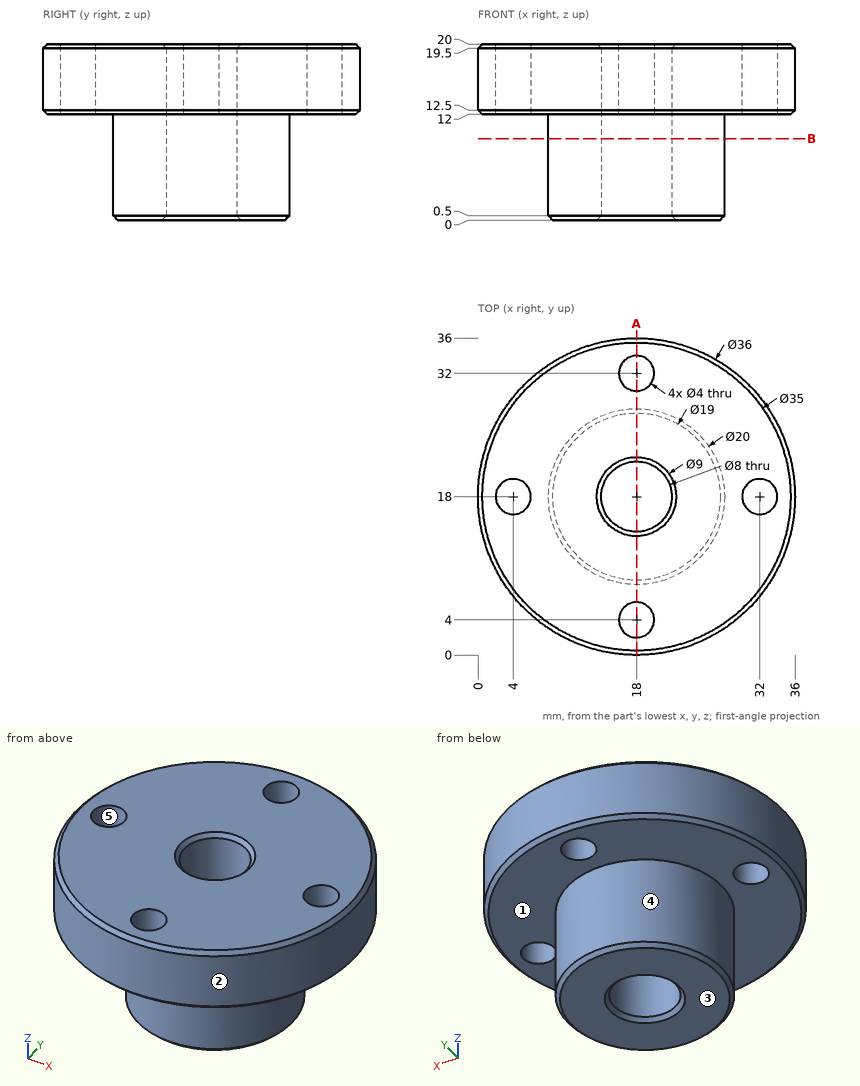
Part print with two shaded views. Sizes in mm from the minimum x, y, z corner. A direction names the side the tool comes from. Round coordinates to 2 decimals unless told otherwise and drop trailing zeros. Write each loop counter-clockwise with the first axis right and the second up, starting at its lowest first coordinate (ties: lowest second). Pieces come first, ordered by that corner, then holes. Notation, with made-up numbers: M -16.75,12.25 L 29.25,12.25 A18 ccw 29.25,45.25 Z; hole C -21,-24.5 d10. An arc over 180 degrees is marked long. Use CSV: the item, a comma, the result in double quotes.
1. Saw through at A-A (x = 18). State how many separate pieces and enclosed holes the cut face has, plus the area to 3 significant figures.
Reply:
separate pieces,"4"
enclosed holes,"0"
area,"303 mm²"
2. Two-plate mould, pull along X, no slides. Class the marked faces 3, 4 and 5: +X half, -X half, draft (parallel to the pull), parting line (faces both ways), or undercut.
Reply:
face 3,"draft"
face 4,"parting line"
face 5,"undercut"
3. Wall check: probe 1 along Y at (x, z) = (18, 13.75); probe 2 along X at (y, z) = (18, 6); probe 3 along Y at (x, z) = (18, 12.25). Give the ranges that are in metal, low to high. Write a range as from..to.
Reply:
probe 1,"y = 0..2, 6..14, 22..30, 34..36"
probe 2,"x = 8..14, 22..28"
probe 3,"y = 0.25..2, 6..14, 22..30, 34..35.75"
4. Saw through at B-B (z = 9.25). Give the cut face in (x, y), plus the area to 3 significant figures.
Reply:
outline,"C 18,18 d20; hole C 18,18 d8"
area,"264 mm²"
5. Tool access for the marked faces 1 and 2: list every direction of +Z, -Z, +X, -X, +Y, -Y with a clear straight run to the whole face (end or side of a thin tool).
Reply:
face 1,"-Z"
face 2,"+Z, -Z"
6. Flat gauge pins, fed straight in: pin 1 (10.5 mm diameter, centred on x = 18, y = 18, fed in from -Z); pin 2 (5 mm diameter, centred on y = 8.5, z = 12.5, fed in from +X); pin 3 (8 mm diameter, centred on x = 7.5, z = 7, fed in from +Y); pin 4 (5 mm diameter, centred on x = 18, y = 4, fed in from -Z). Where does each tip first touch, or does it go through?
Reply:
pin 1,"stops at z = 0"
pin 2,"stops at x = 34.58"
pin 3,"stops at y = 25.6"
pin 4,"stops at z = 12"
